Work out the finished part from the listing and answer in its coordinate system (mm). Give positions to 0.01 mm unless a question says otherwise; leave off trailing zeros. Order: outer loops, then holes, each group sorted by start corner. A loop starts at its lowest first (then second) coordinate and runs counter-clockwise, first axis right, second up. Notation, with made-up numbers: (49, 57.5) - (105, 57.5) arc R13 cw to (105, 73.5) - close; hole circle Ø1 at (57.25, 89.5). An arc over 180 degrees is marked (long way). Return JSON: item names as keys, results as strings. Group by question number.
Autodesk Fusion 360 part; units mm, degrees
sketch "スケッチ1" plane through (0, 0, 0) normal (0, 1, 0) x (1, 0, 0)
  line L0 (-132, 0) -> (132, 0)
  line L1 (-132, 0) -> (-132, -10)
  line L2 (-132, -10) -> (-128, -10)
  line L3 (-128, -10) -> (-128, -20)
  line L4 (-128, -20) -> (-132, -20)
  line L5 (-132, -20) -> (-132, -30)
  line L6 (-132, -30) -> (-128, -30)
  line L7 (-128, -30) -> (-128, -40)
  line L8 (-128, -40) -> (-132, -40)
  line L9 (-132, -40) -> (-132, -50)
  line L10 (-132, -50) -> (132, -50)
  line L11 (132, 0) -> (132, -10)
  line L12 (132, -10) -> (128, -10)
  line L13 (128, -10) -> (128, -20)
  line L14 (128, -20) -> (132, -20)
  line L15 (132, -20) -> (132, -30)
  line L16 (132, -30) -> (128, -30)
  line L17 (128, -30) -> (128, -40)
  line L18 (128, -40) -> (132, -40)
  line L19 (132, -40) -> (132, -50)
  line L20 (-78, 0) -> (-62, 0)
  line L21 (-62, 0) -> (-62, -10)
  line L22 (-62, -10) -> (-78, -10)
  line L23 (-78, -10) -> (-78, 0)
  line L24 (62, 0) -> (78, 0)
  line L25 (78, 0) -> (78, -10)
  line L26 (78, -10) -> (62, -10)
  line L27 (62, -10) -> (62, 0)
  line L28 (-113, -55) -> (-97, -55)
  line L29 (-97, -55) -> (-97, -50)
  line L30 (-97, -50) -> (-113, -50)
  line L31 (-113, -50) -> (-113, -55)
  line L32 (97, -55) -> (113, -55)
  line L33 (113, -55) -> (113, -50)
  line L34 (113, -50) -> (97, -50)
  line L35 (97, -50) -> (97, -55)
  line L36 (-90, -50) -> (-63, -50)
  line L37 (-63, -50) -> (-63, -38)
  line L38 (-63, -38) -> (-90, -38)
  line L39 (-90, -38) -> (-90, -50)
  line L40 (90, -50) -> (75, -50)
  line L41 (75, -50) -> (75, -42)
  line L42 (75, -42) -> (90, -42)
  line L43 (90, -42) -> (90, -50)
  point P0 (0, -25)
  point P1 (-105, -50)
  point P2 (105, -50)
  dimension "d1" = 264
  dimension "d2" = 10
  dimension "d3" = 10
  dimension "d4" = 10
  dimension "d5" = 10
  dimension "d6" = 10
  dimension "d7" = 4
  dimension "d9" = 4
  dimension "d40" = 62
  dimension "d41" = 16
  dimension "d42" = 10
  dimension "d43" = 62
  dimension "d45" = 5
  dimension "d46" = 16
  dimension "d47" = 105
  dimension "d48" = 105
  dimension "d51" = 63
  dimension "d52" = 27
  dimension "d53" = 12
  dimension "d54" = 75
  dimension "d55" = 15
  dimension "d56" = 8
extrude "押し出し1" add sketch "スケッチ1" along normal blind 4 contours L0 L1 L2 L3 L4 L5 L6 L7 L8 L9 L10 L11 L12 L13 L14 L15 L16 L17 L18 L19 L21 L22 L23 L25 L26 L27 L30 L34 L37 L38 L39 L41 L42 L43 | L10 L28 L29 L30 L31 | L10 L32 L33 L34 L35
sketch "スケッチ2" plane through (0, 4, 0) normal (0, 1, 0) x (-1, 0, 0)
  line L0 (-132, 50) -> (-132, 40)
  line L1 (-132, 40) -> (-128, 40)
  line L2 (-128, 40) -> (-128, 30)
  line L3 (-128, 30) -> (-132, 30)
  line L4 (-132, 30) -> (-132, 20)
  line L5 (-132, 20) -> (-128, 20)
  line L6 (-128, 20) -> (-128, 10)
  line L7 (-128, 10) -> (-132, 10)
  line L8 (-132, 10) -> (-132, 0)
  line L9 (-62, 0) -> (62, 0)
  line L10 (123, 25) -> (-123, 25)
  line L11 (105, 36.5) -> (-105, 36.5)
  line L12 (132, 0) -> (132, 10)
  line L13 (132, 10) -> (128, 10)
  line L14 (128, 10) -> (128, 20)
  line L15 (128, 20) -> (132, 20)
  line L16 (132, 20) -> (132, 30)
  line L17 (132, 30) -> (128, 30)
  line L18 (128, 30) -> (128, 40)
  line L19 (128, 40) -> (132, 40)
  line L20 (132, 40) -> (132, 50)
  line L21 (63, 50) -> (-75, 50)
  line L22 (-78, 0) -> (-78, 10)
  line L23 (-78, 10) -> (-62, 10)
  line L24 (-62, 10) -> (-62, 0)
  line L25 (62, 0) -> (62, 10)
  line L26 (62, 10) -> (78, 10)
  line L27 (78, 10) -> (78, 0)
  line L28 (78, 0) -> (132, 0)
  line L29 (-132, 0) -> (-78, 0)
  line L30 (113, 50) -> (113, 55)
  line L31 (113, 55) -> (97, 55)
  line L32 (97, 55) -> (97, 50)
  line L33 (97, 50) -> (90, 50)
  line L34 (-97, 50) -> (-97, 55)
  line L35 (-97, 55) -> (-113, 55)
  line L36 (-113, 55) -> (-113, 50)
  line L37 (-113, 50) -> (-132, 50)
  line L38 (-75, 50) -> (-75, 42)
  line L39 (-75, 42) -> (-90, 42)
  line L40 (-90, 42) -> (-90, 50)
  line L41 (-90, 50) -> (-97, 50)
  line L42 (132, 50) -> (113, 50)
  line L43 (90, 50) -> (90, 38)
  line L44 (90, 38) -> (63, 38)
  line L45 (63, 38) -> (63, 50)
  point P0 (0, 5)
  dimension "d17" = 25
  dimension "d19" = 5
  dimension "d24" = 105
  dimension "d25" = 105
  dimension "d44" = 5
  dimension "d49" = 13.5
  dimension "d50" = 5
hole "穴1" at (-123, 4, 25) at (123, 4, 25) at (-105, 4, 36.5) at (105, 4, 36.5) at (0, 4, 5) direction (0, -1, 0) diameter 3.2 end through all
1. Each of these flat-tipped pins is pushed along its axis until it touches: pin 1 (2 mm diameter, centred on x = -119.5, y = 3, fed in from +Z); pin 2 (1 mm diameter, centred on y = 2, z = 38, fed in from +X). Where does it stop, or does it pass through?
2. The part is cut by section A-A (y = 3). State how many separate pieces and enclosed holes the cut face has, and give its area (3 significant figures).
3. The part is cut by section B-B (x = 9.5). Give the vertices of the cut face in (y, z).
4. Consider probe 1 along X at (y, z) = (3.65, 45); probe 2 along X at (y, z) = (1.25, 5); probe 3 along X at (y, z) = (3.15, 36.5). Determine where each line is inside the solid, lowest interval first. Write a range as from..to.
Answers:
{
 "1": {"pin 1": "stops at z = 50", "pin 2": "stops at x = 128"},
 "2": {"separate pieces": "1", "enclosed holes": "5", "area": "12,400 mm^2"},
 "3": {"outline": "(0, 0) - (4, 0) - (4, 50) - (0, 50) - close"},
 "4": {"probe 1": "x = -132..-90, -63..75, 90..132", "probe 2": "x = -132..-78, -62..-1.6, 1.6..62, 78..132", "probe 3": "x = -128..-106.6, -103.4..103.4, 106.6..128"}
}
